Verification items for the finished model (mm, model axes). A direction names the side the tool comes from. Round coordinates to 2 decimals unless told otherwise and drop trailing zeros. Order: outer loops, then holes, each group sorted by start corner. A loop starts at its lowest first (then second) coordinate and runs counter-clockwise, first axis right, second up. Notation, with made-up numbers: (26.5, -7.75) -> (58.5, -7.75) arc R19 ccw to (58.5, 10.25) -> close; hole circle Ø7 at (-13.75, 81.5). An arc over 180 degrees is marked (long way). Return JSON: item names as keys, results as strings. Group by question number.
1) Draft check along X on faces 3 (the flat face through (0, 5, 0)), 4 (the flat face through (-26.486, -6, 6)), 5 (the cylindrical face through (-17.598, -3.328, 10.568)), 6 (the cylindrical face through (-26.507, 7.91, -10.316)). Enter one of: pulls with the +X half, pulls with the -X half, needs draft (parallel to the pull), parting line crosses it, or undercut.
2) Tool access check on faces 1 (the cylindrical face through (-2.35, 0.75, -7.99)), 2 (the flat face through (-27, 5, 0)). Record the directions out of +Z, -Z, +X, -X, +Y, -Y that give a thin tool (end or side, any length) a straight path to the whole face; none if there is none.
3) Section check B-B on y = 0. State how many separate pieces and enclosed holes the cut face has, plus the area to 3 significant figures.
4) Scan lines: L1, parallel to Y at x = -12, z = 0; L2, parallel to Y at x = -7, z = 0. Record each from-to range of solid material in increasing order.
5) Section check C-C on x = -10.5. Enter the section's corners in (y, z), plus the area to 3 significant figures.
6) Depth check by flat-ended pin: pin 1 (8 mm diameter, centred on x = -16, y = -7, fed in from -Z); pin 2 (5 mm diameter, centred on x = -5.5, y = 5, fed in from -Z); pin 3 (4 mm diameter, centred on x = -7, y = -10, fed in from -Z). Enter the tip coordinate at first touch or a pass-through.
```python
from build123d import *

# Parameters (mm, degrees)
F2_SIZE  = 0.5
F4_D     = 5
F4_DEPTH = 13.001


with BuildPart() as f1:
    # F0 (on Front) → F1 (revolve)
    with BuildSketch(Plane.XZ):
        Polygon((-8.9710751011, 13), (-9.4855375505, 11.08), (-25.4855375505, 11.08), (-26, 13), (-27, 13), (-26.4855375505, 11.08), (-26.4855375505, 8), (-27, 8), (-27, 4), (0, 4), (0, 13), align=None)
    revolve(axis=Axis((-13.5, 0, 0), (1, 0, 0)))

    # F2
    f2_edges = [f1.edges().sort_by_distance(p)[0] for p in [
        (0, 0, -4),
        (0, 0, -13),
        (-27, 0, -8),
        (-27, 0, -4),
    ]]
    chamfer(f2_edges, length=F2_SIZE)

    # F4 (through all, one way)
    with BuildSketch(Plane.XY):
        with Locations((-4.7355375505, 0)):
            Circle(F4_D / 2)
    extrude(amount=-F4_DEPTH, mode=Mode.SUBTRACT)


solid = f1.part
```
Check result:
{
 "1": {"face 3": "pulls with the +X half", "face 4": "pulls with the -X half", "face 5": "undercut", "face 6": "needs draft"},
 "2": {"face 1": "-Z", "face 2": "+Z, -Z, -X, +Y, -Y"},
 "3": {"separate pieces": "3", "enclosed holes": "0", "area": "372 mm^2"},
 "4": {"L1": "-11.08 to -4, 4 to 11.08", "L2": "-13 to -4, 4 to 13"},
 "5": {"outline": "circle Ø22.16 at (0, 0); hole circle Ø8 at (0, 0)", "area": "335 mm^2"},
 "6": {"pin 1": "z = -10.67", "pin 2": "z = -12.76", "pin 3": "z = -10.25"}
}
